Check sheet for the modelled part. Datum: model origin and axes. Units: mm. Face numbers are marked on the shaded views. A direction names the side the tool comes from. Round coordinates to 2 decimals unless told otherwise and drop trailing zeros. Write each loop counter-clockwise with the first axis right and the second up, starting at its lowest first coordinate (ties: lowest second). Pieces come first, ordered by that corner, then holes. Notation, with made-up numbers: (-23, 61) -> (-16, 61) arc R14 ccw to (-16, 66) -> close; hole circle Ø7 at (63, -0.75). An arc over 180 degrees is marked (long way). Use one line per item in the form item = value. Start each with the question number.
```python
from build123d import *

# Parameters (mm, degrees)
F0_W     = 38.1
F0_H     = 63.5
F1_DEPTH = 279.4
F3_DEPTH = 38.101
F4_R     = 6.35
F5_DEPTH = 12.7
F6_R     = 3.175
F7_DEPTH = 50.801


with BuildPart() as f1:
    # F0 (on Right) → F1 (new body, symmetric)
    with BuildSketch(Plane.YZ):
        Rectangle(F0_W, F0_H)
    extrude(amount=F1_DEPTH, both=True)

    # F2 (on face) → F3 (cut, through all)
    with BuildSketch(Plane.XZ.offset(19.05)):
        with BuildLine():
            ThreePointArc((254, 0), (271.960512, -7.439488), (279.4, -25.4))
            Line((279.4, -25.4), (279.4, 31.75))
            Line((279.4, 31.75), (185.42, 31.75))
            ThreePointArc((185.42, 31.75), (196.186422, 27.276422), (200.66, 16.51))
            Line((200.66, 16.51), (200.66, 15.24))
            ThreePointArc((200.66, 15.24), (205.123693, 4.463693), (215.9, 0))
            Line((215.9, 0), (254, 0))
        make_face()
    extrude(amount=-F3_DEPTH, mode=Mode.SUBTRACT)

    # F4 (on face) → F5 (cut)
    with BuildSketch(Plane(origin=(0, 0, -31.75), x_dir=(1, 0, 0), z_dir=(0, 0, -1))):
        with Locations((-260.35, 0)):
            Circle(F4_R)
        with Locations((158.75, 0)):
            Circle(F4_R)
    extrude(amount=-F5_DEPTH, mode=Mode.SUBTRACT)

    # F6 (on face) → F7 (cut, through all)
    with BuildSketch(Plane(origin=(0, 0, -19.05), x_dir=(1, 0, 0), z_dir=(0, 0, -1))):
        with Locations((-260.35, 0)):
            Circle(F6_R)
        with Locations((158.75, 0)):
            Circle(F6_R)
    extrude(amount=-F7_DEPTH, mode=Mode.SUBTRACT)


solid = f1.part
```
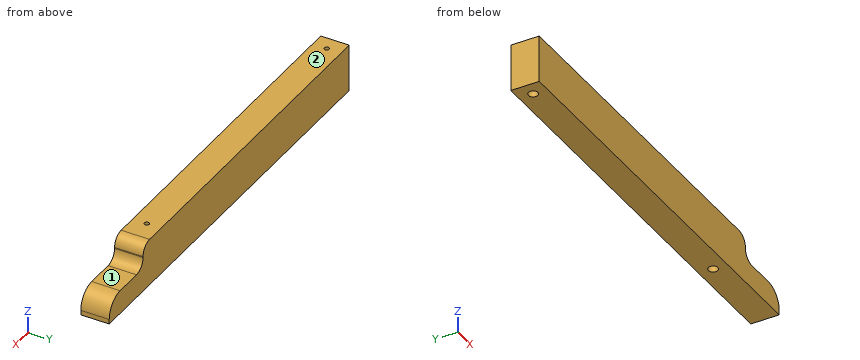
1. Tool access check on the marked faces 1 and 2. Record the directions out of +Z, -Z, +X, -X, +Y, -Y that give a thin tool (end or side, any length) a straight path to the whole face; none if there is none.
2. Sectioned sample at B-B (z = 25.5). Enter the section's corners in (x, y) (3 decimals), and give its area (3 significant figures).
3. Sectioned sample at A-A (y = -14.5). Enter the section's corners in (x, z), and give its area (3 significant figures).
4. Scan lines: probe 1 along X at (y, z) = (0, -28); probe 2 along Y at (x, z) = (-260.35, 1) (3 decimals); probe 3 along Y at (x, z) = (-260.35, -28). Record each from-to range of solid material in increasing order.
5. Depth check by flat-ended pin: pin 1 (8.5 mm diameter, centred on x = -260.35, y = 0, fed in from -Z); pin 2 (0.6 mm diameter, centred on y = 3, z = 16, fed in from +X); pin 3 (4 mm diameter, centred on x = 158.75, y = 0, fed in from -Z). Enter the tip coordinate at first touch or a pass-through.
6. Sectioned sample at C-C (z = 5). Enter the section's corners in (x, y) (3 decimals), and give its area (3 significant figures).
Returned:
q1.face_1 = +Z, +X, +Y, -Y
q1.face_2 = +Z, +X, -X, +Y, -Y
q2.outline = (-279.4, -19.05) -> (197.709, -19.05) -> (197.709, 19.05) -> (-279.4, 19.05) -> close; hole circle Ø6.35 at (-260.35, 0); hole circle Ø6.35 at (158.75, 0)
q2.area = 18,100 mm^2
q3.outline = (-279.4, -31.75) -> (279.4, -31.75) -> (279.4, -25.4) arc R25.4 ccw to (254, 0) -> (215.9, 0) arc R15.24 cw to (200.66, 15.24) -> (200.66, 16.51) arc R15.27 ccw to (185.42, 31.75) -> (-279.4, 31.75) -> close
q3.area = 32,800 mm^2
q4.probe_1 = -279.4 to -266.7, -254 to 152.4, 165.1 to 279.4
q4.probe_2 = -19.05 to -3.175, 3.175 to 19.05
q4.probe_3 = -19.05 to -6.35, 6.35 to 19.05
q5.pin_1 = -19.05
q5.pin_2 = 200.66
q5.pin_3 = through
q6.outline = (-279.4, -19.05) -> (204.613, -19.05) -> (204.613, 19.05) -> (-279.4, 19.05) -> close; hole circle Ø6.35 at (-260.35, 0); hole circle Ø6.35 at (158.75, 0)
q6.area = 18,400 mm^2
